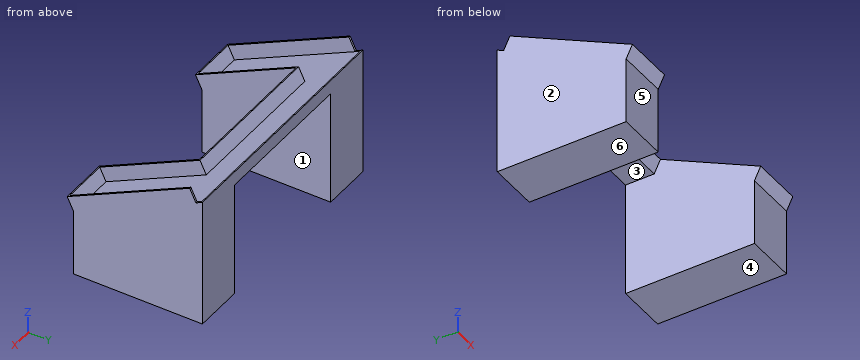
from build123d import *

# Parameters (mm, degrees)
F1_DEPTH = 889
F2_W     = 533.4
F2_H     = 235.7679336681
F2_H_2   = 224.7003448227
F3_DEPTH = 355.6
F5_DEPTH = 50.8
F6_DEPTH = 25.4
F7_DEPTH = 101.601


with BuildPart() as f1:
    # F0 (on Right) → F1 (new body)
    with BuildSketch(Plane.YZ):
        Polygon((0, -235.7679336681), (0, 221.4320663319), (-457.2, 0), (-457.2, -235.7679336681), align=None)
    extrude(amount=F1_DEPTH)

    # F2 (on face) → F3 (cut)
    with BuildSketch(Plane.XZ.offset(457.2)):
        with Locations((444.5, -117.8839668341)):
            Rectangle(F2_W, F2_H)
        with Locations((444.5, 112.3501724113)):
            Rectangle(F2_W, F2_H_2)
    extrude(amount=-F3_DEPTH, mode=Mode.SUBTRACT)

    # F4 (on face) → F5 (join)
    with BuildSketch(Plane(origin=(0, -86.868, 179.3599737288), x_dir=(1, 0, 0), z_dir=(0, -0.4358898944, 0.9))):
        Polygon((889, 96.52), (0, 96.52), (0, -411.48), (177.8, -411.48), (177.8, -16.3688888889), (711.2, -16.3688888889), (711.2, -411.48), (889, -411.48), align=None)
        Polygon((6.35, -405.13), (6.35, 90.17), (882.65, 90.17), (882.65, -405.13), (717.55, -405.13), (717.55, -10.0188888889), (171.45, -10.0188888889), (171.45, -405.13), align=None, mode=Mode.SUBTRACT)
    extrude(amount=F5_DEPTH)

    # F6 (cut): a face of the model
    f6_faces = [f1.faces().sort_by_distance(p)[0] for p in [
        (444.5, -11.0716033166, 244.2920663319),
    ]]
    extrude(f6_faces, amount=-F6_DEPTH, mode=Mode.SUBTRACT)

    # F7 (cut, through all): a face of the model
    f7_faces = [f1.faces().sort_by_distance(p)[0] for p in [
        (444.5, -101.6, -31.7714965939),
    ]]
    extrude(f7_faces, amount=-F7_DEPTH, mode=Mode.SUBTRACT)


solid = f1.part
The model under review builds one solid part; all positions refer to its coordinate system, in mm. Face numbers are marked on the shaded views. A direction names the side the tool comes from. Round coordinates to 2 decimals unless told otherwise and drop trailing zeros. Loops run counter-clockwise (first coordinate to the right, second up) from the corner with the lowest first, then second, coordinate; pieces in that order, holes last. Notation, with made-up numbers: (-1.75, -31) -> (48.25, -31) arc R27 cw to (48.25, 6) -> close; hole circle Ø11 at (40.25, 50). An arc over 180 degrees is marked (long way). Answer as CSV lines item,"result".
1) Add section B-B on y = -310.5. Write out the cut boundary in (x, z), plus the area to 3 significant figures.
Geometry results:
outline,"(0, -235.77) -> (177.8, -235.77) -> (177.8, 127.49) -> (171.45, 127.49) -> (171.45, 71.05) -> (6.35, 71.05) -> (6.35, 127.49) -> (0, 127.49) -> close; (711.2, -235.77) -> (889, -235.77) -> (889, 127.49) -> (882.65, 127.49) -> (882.65, 71.05) -> (717.55, 71.05) -> (717.55, 127.49) -> (711.2, 127.49) -> close"
area,"111,000 mm²"
2) Add section A-A on z = -164. Write out the cut boundary in (x, y), plus the area to 3 significant figures.
Geometry results:
outline,"(0, -457.2) -> (177.8, -457.2) -> (177.8, 0) -> (0, 0) -> close; (711.2, -457.2) -> (889, -457.2) -> (889, 0) -> (711.2, 0) -> close"
area,"163,000 mm²"
3) To check wall thickness, follow line 1 along X through (y, z) = (-213, 141); line 2 along X through (y, z) = (-337, -37.5); line 3 along Y through (x, z) = (691, 210.5). State the ranges of each line that lie inside material, in increasing order. Write a range as from..to.
Geometry results:
line 1,"x = 0..6.35, 171.45..177.8, 711.2..717.55, 882.65..889"
line 2,"x = 0..177.8, 711.2..889"
line 3,"y = -120.14..-113.08, -22.57..0"
4) For P1, Ø10, axis at x = 760, y = -161.5, coming from the +Z side, flat-tipped, find the tip position at first contact; note if it passes through.
Geometry results:
P1,"stops at z = 145.64"
5) Draft analysis for pull direction X (two halves, no side actions). For the marked faces 1, 2, 3 and 4, state which applies: pulls with the +X half, pulls with the -X half, needs draft (parallel to the pull), parting line crosses it, or undercut.
Geometry results:
face 1,"undercut"
face 2,"pulls with the -X half"
face 3,"undercut"
face 4,"needs draft"
6) Tool access review of the marked faces 5 and 6: name each direction out of +Z, -Z, +X, -X, +Y, -Y from which nothing blocks a thin tool from reaching the whole face with its end or side.
Geometry results:
face 5,"-Z, +X, -X, -Y"
face 6,"-Z, +X, -X, +Y, -Y"
7) Add section C-C on x = 480.5. Write out the cut boundary in (y, z) (3 decimals), plus the area to 3 significant figures.
Geometry results:
outline,"(-123.743, 217.945) -> (-101.6, 172.225) -> (0, 172.225) -> (0, 221.432) -> (-95.885, 174.993) -> (-118.028, 220.713) -> close"
area,"2,820 mm²"
8) Add section D-D on z = 163. Write out the cut boundary in (x, y).
Geometry results:
outline,"(0, -237.19) -> (6.35, -237.19) -> (6.35, -120.65) -> (171.45, -120.65) -> (171.45, -237.19) -> (177.8, -237.19) -> (177.8, 0) -> (0, 0) -> close; (711.2, -237.19) -> (717.55, -237.19) -> (717.55, -120.65) -> (882.65, -120.65) -> (882.65, -237.19) -> (889, -237.19) -> (889, 0) -> (711.2, 0) -> close"
